Geometry: final body of the model. Coordinates: model frame, mm. Face numbers are marked on the shaded views. A direction names the side the tool comes from. Round coordinates to 2 decimals unless told otherwise and drop trailing zeros. Order: outer loops, then holes, each group sorted by start corner. A loop starts at its lowest first (then second) coordinate and runs counter-clockwise, first axis right, second up. Notation, with made-up numbers: (65.25, -9) -> (102.25, -9) arc R14 ccw to (102.25, 8) -> close; hole circle Ø11 at (18.5, 63.5). An arc over 180 degrees is marked (long way). Put each result on its own line as item: value.
```python
from build123d import *

# Parameters (mm, degrees)
SKETCH1_R           = 5
BOSS_EXTRUDE1_DEPTH = 15
CUT_EXTRUDE1_START  = -15
CUT_EXTRUDE1_DEPTH  = 15
BOSS_EXTRUDE2_START = -15
BOSS_EXTRUDE2_DEPTH = 15
FILLET1_R           = 10


with BuildPart() as part:
    # Sketch1 → Boss-Extrude1 (new body)
    with BuildSketch(Plane.XY):
        with BuildLine():
            Line((0, 0), (-10, 0))
            Line((-10, 0), (-48.033043506, -60))
            Line((-48.033043506, -60), (-30, -105))
            ThreePointArc((-30, -105), (-1.41305071, -111.355691072), (-24.614025467, -93.486073028))
            Line((-24.614025467, -93.486073028), (-36.029372005, -65))
            Line((-36.029372005, -65), (0, -65))
            Line((0, -65), (0, 0))
        make_face()
        Polygon((-5, -50), (-5, -60), (-43.033043506, -60), (-36.694202922, -50), align=None, mode=Mode.SUBTRACT)
        Polygon((-27.185942045, -35), (-5, -35), (-5, -45), (-33.52478263, -45), align=None, mode=Mode.SUBTRACT)
        Polygon((-17.677681169, -20), (-5, -20), (-5, -30), (-24.016521753, -30), align=None, mode=Mode.SUBTRACT)
        Polygon((-14.508260877, -15), (-8.169420292, -5), (-5, -5), (-5, -15), align=None, mode=Mode.SUBTRACT)
        with Locations((-15, -105)):
            Circle(SKETCH1_R, mode=Mode.SUBTRACT)
    extrude(amount=BOSS_EXTRUDE1_DEPTH)

    # Sketch2 → Cut-Extrude1 (cut)
    with BuildSketch(Plane.XY.offset(15).offset(CUT_EXTRUDE1_START)):
        with BuildLine():
            Line((-15, -90), (-15, -92.5))
            ThreePointArc((-15, -92.5), (-3.506810704, -109.914936399), (-24.038127106, -113.634944031))
            Line((-24.038127106, -113.634944031), (-25.845752528, -115.361932837))
            ThreePointArc((-25.845752528, -115.361932837), (-1.208172845, -110.897923679), (-15, -90))
        make_face()
    extrude(amount=CUT_EXTRUDE1_DEPTH, mode=Mode.SUBTRACT)

    # Sketch3 → Boss-Extrude2 (add)
    with BuildSketch(Plane.XY.offset(15).offset(BOSS_EXTRUDE2_START)):
        with BuildLine():
            Line((-14.5, -90), (-15, -90))
            Line((-15, -90), (-15, -92.5))
            ThreePointArc((-15, -92.5), (-14.279138, -92.520802992), (-13.560675373, -92.583142724))
            Line((-13.560675373, -92.583142724), (-14.5, -90))
        make_face()
        with BuildLine():
            Line((-10.840273343, -90.579643758), (-12.53185915, -92.746091205))
            ThreePointArc((-12.53185915, -92.746091205), (-11.13728757, -93.111793546), (-9.79410102, -93.635642746))
            Line((-9.79410102, -93.635642746), (-9.889216826, -90.888660753))
            Line((-9.889216826, -90.888660753), (-10.840273343, -90.579643758))
        make_face()
        with BuildLine():
            Line((-6.587729713, -92.570852458), (-8.865992497, -94.108537658))
            ThreePointArc((-8.865992497, -94.108537658), (-7.652684346, -94.88728757), (-6.53711633, -95.800565236))
            Line((-6.53711633, -95.800565236), (-5.778712718, -93.158637711))
            Line((-5.778712718, -93.158637711), (-6.587729713, -92.570852458))
        make_face()
        with BuildLine():
            Line((-3.158637711, -95.778712718), (-5.800565236, -96.53711633))
            ThreePointArc((-5.800565236, -96.53711633), (-4.88728757, -97.652684346), (-4.108537658, -98.865992497))
            Line((-4.108537658, -98.865992497), (-2.570852458, -96.587729713))
            Line((-2.570852458, -96.587729713), (-3.158637711, -95.778712718))
        make_face()
        with BuildLine():
            Line((-0.888660753, -99.889216826), (-3.635642746, -99.79410102))
            ThreePointArc((-3.635642746, -99.79410102), (-3.111793546, -101.13728757), (-2.746091205, -102.53185915))
            Line((-2.746091205, -102.53185915), (-0.579643758, -100.840273343))
            Line((-0.579643758, -100.840273343), (-0.888660753, -99.889216826))
        make_face()
        with BuildLine():
            Line((0, -104.5), (-2.583142724, -103.560675373))
            ThreePointArc((-2.583142724, -103.560675373), (-2.5, -105), (-2.583142724, -106.439324627))
            Line((-2.583142724, -106.439324627), (0, -105.5))
            Line((0, -105.5), (0, -104.5))
        make_face()
        with BuildLine():
            Line((-0.579643758, -109.159726657), (-2.746091205, -107.46814085))
            ThreePointArc((-2.746091205, -107.46814085), (-3.111793546, -108.86271243), (-3.635642746, -110.20589898))
            Line((-3.635642746, -110.20589898), (-0.888660753, -110.110783174))
            Line((-0.888660753, -110.110783174), (-0.579643758, -109.159726657))
        make_face()
        with BuildLine():
            ThreePointArc((-21.134007503, -115.891462342), (-22.347315654, -115.11271243), (-23.46288367, -114.199434764))
            Line((-23.46288367, -114.199434764), (-24.221287282, -116.841362289))
            Line((-24.221287282, -116.841362289), (-23.412270287, -117.429147542))
            Line((-23.412270287, -117.429147542), (-21.134007503, -115.891462342))
        make_face()
        with BuildLine():
            Line((-2.570852458, -113.412270287), (-4.108537658, -111.134007503))
            ThreePointArc((-4.108537658, -111.134007503), (-4.88728757, -112.347315654), (-5.800565236, -113.46288367))
            Line((-5.800565236, -113.46288367), (-3.158637711, -114.221287282))
            Line((-3.158637711, -114.221287282), (-2.570852458, -113.412270287))
        make_face()
        with BuildLine():
            ThreePointArc((-17.46814085, -117.253908795), (-18.86271243, -116.888206454), (-20.20589898, -116.364357254))
            Line((-20.20589898, -116.364357254), (-20.110783174, -119.111339247))
            Line((-20.110783174, -119.111339247), (-19.159726657, -119.420356242))
            Line((-19.159726657, -119.420356242), (-17.46814085, -117.253908795))
        make_face()
        with BuildLine():
            Line((-5.778712718, -116.841362289), (-6.53711633, -114.199434764))
            ThreePointArc((-6.53711633, -114.199434764), (-7.652684346, -115.11271243), (-8.865992497, -115.891462342))
            Line((-8.865992497, -115.891462342), (-6.587729713, -117.429147542))
            Line((-6.587729713, -117.429147542), (-5.778712718, -116.841362289))
        make_face()
        with BuildLine():
            ThreePointArc((-13.560675373, -117.416857276), (-15, -117.5), (-16.439324627, -117.416857276))
            Line((-16.439324627, -117.416857276), (-15.5, -120))
            Line((-15.5, -120), (-14.5, -120))
            Line((-14.5, -120), (-13.560675373, -117.416857276))
        make_face()
        with BuildLine():
            Line((-9.889216826, -119.111339247), (-9.79410102, -116.364357254))
            ThreePointArc((-9.79410102, -116.364357254), (-11.13728757, -116.888206454), (-12.53185915, -117.253908795))
            Line((-12.53185915, -117.253908795), (-10.840273343, -119.420356242))
            Line((-10.840273343, -119.420356242), (-9.889216826, -119.111339247))
        make_face()
    extrude(amount=BOSS_EXTRUDE2_DEPTH)

    # Fillet1
    fillet1_edges = [part.edges().sort_by_distance(p)[0] for p in [
        (-48.033043506, -60, 7.5),
    ]]
    fillet(fillet1_edges, radius=FILLET1_R)


solid = part.part
```
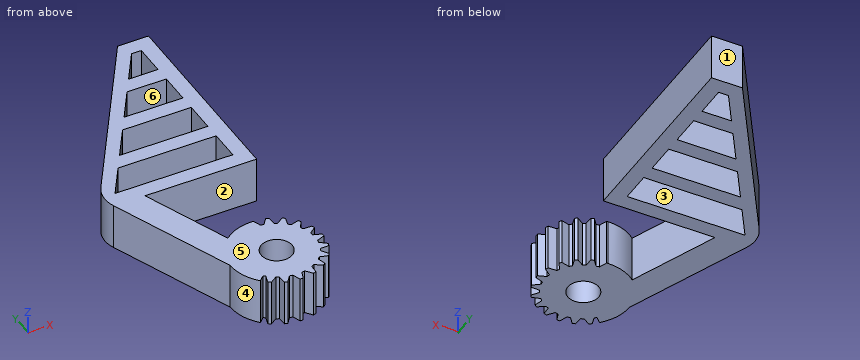
1. Cut plane A-A on x = -28.5. Return loops of the section in (y, z), and give its area (3 significant figures).
Ans:
outline: (-111.54, 0) -> (-83.79, 0) -> (-83.79, 15) -> (-111.54, 15) -> close; (-65, 0) -> (-60, 0) -> (-60, 15) -> (-65, 15) -> close; (-50, 0) -> (-45, 0) -> (-45, 15) -> (-50, 15) -> close; (-37.07, 0) -> (-29.19, 0) -> (-29.19, 15) -> (-37.07, 15) -> close
area: 685 mm²
2. Cut plane B-B on x = -38.5. Return loops of the section in (y, z).
Ans:
outline: (-83.79, 0) -> (-60, 0) -> (-60, 15) -> (-83.79, 15) -> close; (-52.85, 0) -> (-44.96, 0) -> (-44.96, 15) -> (-52.85, 15) -> close
3. Cut plane C-C on z = 13.25. State how many separate pieces and enclosed holes the cut face has, and give its area (3 significant figures).
Ans:
separate pieces: 1
enclosed holes: 5
area: 2,030 mm²
4. Draft query along Y for the marked faces 4, 5 and 6. Return one class per face: +Y half, -Y half, draft (parallel to the pull), parting line (faces both ways), or undercut.
Ans:
face 4: -Y half
face 5: draft
face 6: undercut
5. Set-up query: the marked faces 1, 2 and 3. Return all of +Z, -Z, +X, -X, +Y, -Y with unobstructed straight access to the full face (end or side cutting, diameter ignored); none if empty.
Ans:
face 1: +Z, -Z, +X, -X, +Y
face 2: +Z, -Z, +X
face 3: +Z, -Z
6. Cut plane D-D on y = -78. Return loops of the section in (x, z), and give its area (3 significant figures).
Ans:
outline: (-40.82, 0) -> (-30.82, 0) -> (-30.82, 15) -> (-40.82, 15) -> close
area: 150 mm²
7. Contact query for flat-ended pins moving along their axis: P1, Ø4.5, axis at x = -22, z = 10.5, coming from the +Y side; P2, Ø1, axis at y = -95, z = 12.5, coming from the +X side; P3, Ø4.5, axis at x = -26, z = 4.5, coming from the -Y side. Output: stop coordinate, or through.
Ans:
P1: y = -15.38
P2: x = -6.16
P3: y = -117.18
8. Material intervals for probe 1 along Y at (x, z) = (-31, 13.5); probe 2 along Y at (x, z) = (-7.5, 8.5); probe 3 along Y at (x, z) = (-28.5, 11), sorted ascending.
Ans:
probe 1: -102.5 to -77.55, -65 to -60, -50 to -45, -41.02 to -33.13
probe 2: -116.81 to -93.19, -65 to -60, -50 to -45, -35 to -30, -20 to -15, -5 to 0
probe 3: -111.54 to -83.79, -65 to -60, -50 to -45, -37.07 to -29.19
